Check sheet for the modelled part. Datum: model origin and axes. Units: mm. A direction names the side the tool comes from. Round coordinates to 2 decimals unless told otherwise and drop trailing zeros. Order: outer loops, then holes, each group sorted by start corner. A loop starts at its lowest first (then second) coordinate and runs counter-clockwise, first axis right, second up. Notation, with made-up numbers: (80.5, 33.5) -> (97.5, 33.5) arc R28 cw to (97.5, 72.5) -> close; hole circle Ø9 at (69.5, -3). An arc over 180 degrees is marked (long way). Answer in a Markdown table with one row per item. Add a question column.
1. Depth check by flat-ended pin: P1, Ø1.5, axis at y = -7, z = 26, coming from the -X side; P2, Ø10, axis at y = 10.5, z = 40.5, coming from the +X side; P3, Ø4, axis at x = -4, z = 38, coming from the +Y side; P4, Ø8, axis at y = -19.5, z = 47.5, coming from the -X side. Enter the tip coordinate at first touch or a pass-through.
2. Material ranges on L1, parallel to Z at x = -10, y = -9; L2, parallel to Y at x = 0.5, z = 24; L3, parallel to Y at x = -6.5, z = 45, recorded low to high. Write a range as from..to.
3. Sectioned sample at B-B, the plane z = 57. Record the boundary of the cut face in (x, y).
4. Sectioned sample at C-C, the plane z = 24.5. Record the boundary of the cut face in (x, y).
5. Sectioned sample at A-A, the plane x = 0. Record the boundary of the cut face in (y, z).
6. Draft check along X on faces 1 (the cylindrical face through (-15.12, -11.59, 22.66)), 2 (the flat face through (0, 0, 0)), 3 (the cylindrical face through (4.48, 1.72, 51.93)). Enter one of: +X half, -X half, draft (parallel to the pull), parting line (faces both ways), or undercut.
7. Access from +Z, -Z, +X, -X, +Y, -Y to the whole of each face (thin tool, end or side, straight path). Record for faces 4 (the cylindrical face through (-8.4, -1.5, 51.9)), 5 (the flat face through (6, 0, 62.23)).
```python
from build123d import *

# Parameters (mm, degrees)
F0_R     = 27.94
F1_DEPTH = 3.81
F2_R     = 19.05
F3_DEPTH = 38.1
F4_R     = 5.08
F5_SIZE  = 5.08
F6_R     = 2.54
F7_DEPTH = 20.32


with BuildPart() as f1:
    # F0 (on Top) → F1 (new body)
    with BuildSketch(Plane.XY):
        Circle(F0_R)
    extrude(amount=F1_DEPTH)

    # F2 (on face) → F3 (join)
    with BuildSketch(Plane.XY.offset(3.81)):
        Circle(F2_R)
    extrude(amount=F3_DEPTH)

    # F4
    f4_edges = [f1.edges().sort_by_distance(p)[0] for p in [
        (-19.05, 0, 41.91),
    ]]
    fillet(f4_edges, radius=F4_R)

    # F5
    f5_edges = [f1.edges().sort_by_distance(p)[0] for p in [
        (19.05, 0, 20.32),
        (-19.05, 0, 36.83),
        (-19.05, 0, 3.81),
    ]]
    chamfer(f5_edges, length=F5_SIZE)

    # F6 (on face) → F7 (join)
    with BuildSketch(Plane.XY.offset(41.91)):
        with Locations((-6.35, 0)):
            Circle(F6_R)
        with Locations((6.35, 0)):
            Circle(F6_R)
    extrude(amount=F7_DEPTH)


solid = f1.part
```
Answer key:
| question | item | result |
|---|---|---|
| 1 | P1 | stops at x = -18 |
| 1 | P2 | stops at x = 17.88 |
| 1 | P3 | stops at y = 18.91 |
| 1 | P4 | passes through |
| 2 | L1 | z = 0..41.91 |
| 2 | L2 | y = -19.04..19.04 |
| 2 | L3 | y = -2.54..2.54 |
| 3 | outline | circle Ø5.08 at (-6.35, 0); circle Ø5.08 at (6.35, 0) |
| 4 | outline | circle Ø38.1 at (0, 0) |
| 5 | outline | (-27.94, 0) -> (27.94, 0) -> (27.94, 3.81) -> (24.13, 3.81) -> (19.05, 8.89) -> (19.05, 36.83) arc R5.08 ccw to (13.97, 41.91) -> (-13.97, 41.91) arc R5.08 ccw to (-19.05, 36.83) -> (-19.05, 8.89) -> (-24.13, 3.81) -> (-27.94, 3.81) -> close |
| 6 | face 1 | parting line |
| 6 | face 2 | draft |
| 6 | face 3 | undercut |
| 7 | face 4 | +Z |
| 7 | face 5 | +Z, +X, -X, +Y, -Y |
